Verification items for the finished model (mm, model axes). Face numbers are marked on the shaded views. A direction names the side the tool comes from. Give positions to 0.01 mm unless a question says otherwise; leave off trailing zeros. Write each loop counter-clockwise with the first axis right and the second up, starting at its lowest first coordinate (ties: lowest second). Pieces come first, ordered by that corner, then holes.
from build123d import *

# Parameters (mm, degrees)
BOSS_EXTRUDE1_DEPTH    = 7.9375
F_10_CLEARANCE_HOLE1_D = 5.1054


with BuildPart() as part:
    # Sketch2 → Boss-Extrude1 (new, symmetric)
    with BuildSketch(Plane.XY):
        Polygon((-2.5, 7.9375), (2.5, 7.9375), (22, 7.9375), (22, 2.9375), (2.5, 2.9375), (2.5, -7.9375), (-2.5, -7.9375), align=None)
    extrude(amount=BOSS_EXTRUDE1_DEPTH, both=True)

    # #10 Clearance Hole1 (through all)
    with Locations(Plane(origin=(2.5, 0, 0), x_dir=(0, 0, -1), z_dir=(1, 0, 0))):
        with Locations((0, -1.5625)):
            Hole(F_10_CLEARANCE_HOLE1_D / 2)


solid = part.part
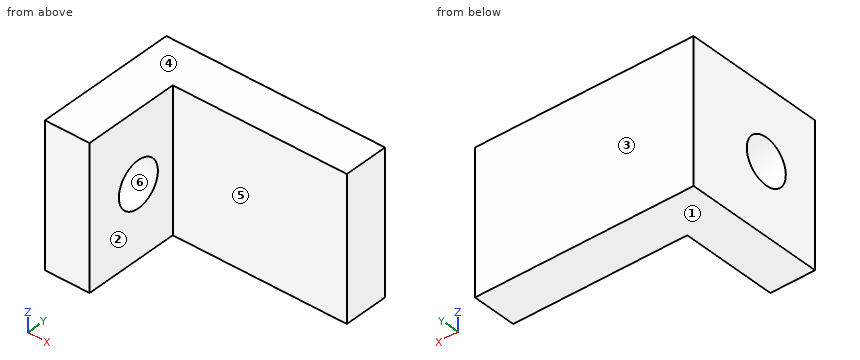
Item 1: Set-up check for the marked faces 1 and 2: record each of +Z, -Z, +X, -X, +Y, -Y from which the full face is reachable in a straight line by a thin tool's end or side.
Answer key:
face 1: -Z, +X, -X, +Y, -Y
face 2: +Z, -Z, +X, -Y
Item 2: Scan lines: line 1 along Y through (x, z) = (0.4, 0); line 2 along X through (y, z) = (-3.75, 2.5); line 3 along Y through (x, z) = (11, -1). Record each from-to range of solid material in increasing order.
Answer key:
line 1: y = -7.94 to -4.12, 0.99 to 7.94
line 2: x = -2.5 to 2.5
line 3: y = 2.94 to 7.94
Item 3: Sectioned sample at A-A on z = 0. Record the cut outline in (x, y), then the cut area to 3 significant figures.
Answer key:
outline: (-2.5, -7.94) - (2.5, -7.94) - (2.5, -4.12) - (-2.5, -4.12) - close; (-2.5, 0.99) - (2.5, 0.99) - (2.5, 2.94) - (22, 2.94) - (22, 7.94) - (-2.5, 7.94) - close
area: 151 mm2
Item 4: Release check for a two-part mould opening along Y. For the marked faces 3, 4, 5 and 6 record: released by +Y, released by -Y, zero draft, split by the parting line, or undercut.
Answer key:
face 3: released by +Y
face 4: zero draft
face 5: released by -Y
face 6: undercut
Item 5: Sectioned sample at B-B on y = -2. Record the cut outline in (x, z).
Answer key:
outline: (-2.5, -7.94) - (2.5, -7.94) - (2.5, -2.51) - (-2.5, -2.51) - close; (-2.5, 2.51) - (2.5, 2.51) - (2.5, 7.94) - (-2.5, 7.94) - close
Item 6: Sectioned sample at D-D on x = 12.25. Record the cut outline in (y, z).
Answer key:
outline: (2.94, -7.94) - (7.94, -7.94) - (7.94, 7.94) - (2.94, 7.94) - close
Item 7: Sectioned sample at C-C on z = -6. Record the cut outline in (x, y), then the cut area to 3 significant figures.
Answer key:
outline: (-2.5, -7.94) - (2.5, -7.94) - (2.5, 2.94) - (22, 2.94) - (22, 7.94) - (-2.5, 7.94) - close
area: 177 mm2
Item 8: Depth check by flat-ended pin: pin 1 (6.5 mm diameter, centred on y = -1.56, z = 0, fed in from +X); pin 2 (6 mm diameter, centred on x = 12, z = -0.5, fed in from -Y). Enter the tip coordinate at first touch or a pass-through.
Answer key:
pin 1: stops at x = 2.5
pin 2: stops at y = 2.94
